Here's how the part is built. I have some questions about the finished solid (model axes, mm). Give positions to 0.01 mm unless a question says otherwise; leave off trailing zeros. Write each loop counter-clockwise with the first axis right and the second up, starting at its lowest first coordinate (ties: lowest second). Pieces come first, ordered by that corner, then holes. Notation, with made-up numbers: (65.25, -34) - (113.25, -34) arc R28 ccw to (113.25, 0) - close; hole circle Ø2 at (-36, 17). An arc over 180 degrees is marked (long way). Use a Markdown table: item, result.
```python
from build123d import *

# Parameters (mm, degrees)
F0_R     = 20
F1_DEPTH = 2000
F3_D     = 10
F4_D     = 10
F5_D     = 10
F6_D     = 10


with BuildPart() as f1:
    # F0 (on Front) → F1 (new body)
    with BuildSketch(Plane.XZ):
        Circle(F0_R)
    extrude(amount=F1_DEPTH)

    # F3 (through all)
    with Locations(Plane.YZ):
        with Locations((-1980, 0)):
            Hole(F3_D / 2)

    # F4 (through all)
    with Locations(Plane(origin=(0, 0, 0), x_dir=(0, 1, 0), z_dir=(-1, 0, 0))):
        with Locations((-1980, 0)):
            Hole(F4_D / 2)

    # F5 (through all)
    with Locations(Plane.YZ):
        with Locations((-20, 0)):
            Hole(F5_D / 2)

    # F6 (through all)
    with Locations(Plane(origin=(0, 0, 0), x_dir=(0, 1, 0), z_dir=(-1, 0, 0))):
        with Locations((-20, 0)):
            Hole(F6_D / 2)


solid = f1.part
```
Item 1: Will these pins go through, and if not, where does the flat tip stop? pin 1 Ø1.5 at (x, y) = (12, -1780.5) entering from -Z; pin 2 Ø3 at (y, z) = (-1088.5, -14.5) entering from -X; pin 3 Ø6 at (y, z) = (-1042, -13.5) entering from -X.
Values:
| item | result |
|---|---|
| pin 1 | stops at z = -16.54 |
| pin 2 | stops at x = -15.2 |
| pin 3 | stops at x = -17.02 |
Item 2: If we section it at C-C, the plane z = -13: Write out the boundary of the cut face in (x, y), plus the area to 3 significant figures.
Values:
| item | result |
|---|---|
| outline | (-15.2, -2000) - (15.2, -2000) - (15.2, 0) - (-15.2, 0) - close |
| area | 60,800 mm2 |
Item 3: If we section it at A-A, the plane y = -658.5: Write out the boundary of the cut face in (x, z), plus the area to 3 significant figures.
Values:
| item | result |
|---|---|
| outline | circle Ø40 at (0, 0) |
| area | 1,260 mm2 |
Item 4: If we section it at B-B, the plane x = 11: Write out the boundary of the cut face in (y, z), plus the area to 3 significant figures.
Values:
| item | result |
|---|---|
| outline | (-2000, -16.7) - (0, -16.7) - (0, 16.7) - (-2000, 16.7) - close; hole circle Ø10 at (-1980, 0); hole circle Ø10 at (-20, 0) |
| area | 66,700 mm2 |
Item 5: I need wall thicknesses on line 1 along Y through (x, z) = (-1, 0); line 2 along Z through (x, y) = (2.5, -1980); line 3 along Y through (x, z) = (10.5, 3). Which ranges of each line are inside material? Lowest first, please. Write a range as [from, to].
Values:
| item | result |
|---|---|
| line 1 | y = [-2000, -1985], [-1975, -25], [-15, 0] |
| line 2 | z = [-19.84, -5], [5, 19.84] |
| line 3 | y = [-2000, -1984], [-1976, -24], [-16, 0] |
